from build123d import *

# Parameters (mm, degrees)
SKETCH_2_R                       = 28.3
EXTRUDE_1_DEPTH                  = 1.2
CUT_EXTRUDE_1_DEPTH              = 41.04022977
FILLET_1_R                       = 2
FILLET_2_R                       = 0.2
PATTERN_CIRCULAR_2_COUNT         = 6
FILLET_1_OF_PATTERN_CIRCULAR_2_R = 2
FILLET_2_OF_PATTERN_CIRCULAR_2_R = 0.2
SKETCH_4_R                       = 1.25
SKETCH_4_R_2                     = 1.5
CUT_EXTRUDE_2_DEPTH              = 40.283043416
CUT_EXTRUDE_START                = -1.2
CUT_EXTRUDE_4_DEPTH              = 1.2
SKETCH_7_W                       = 2.25
SKETCH_7_H                       = 2.05
EXTRUDE_2_DEPTH                  = 1.2
SKETCH_8_R                       = 1.3
CUT_EXTRUDE_6_DEPTH              = 1.2
CUT_EXTRUDE_7_DEPTH              = 1.2
FILLET_4_R                       = 1


with BuildPart() as part:
    # ｽｹｯﾁ2 → ﾎﾞｽ - 押し出し1 (new body)
    with BuildSketch(Plane.XY):
        Circle(SKETCH_2_R)
    extrude(amount=EXTRUDE_1_DEPTH)

    # ｽｹｯﾁ3 → ｶｯﾄ - 押し出し1 (cut, through all)
    with BuildSketch(Plane.XY.offset(1.2)):
        Polygon((-7.75, 30.775), (7.75, 30.775), (7.75, 24.3), (10, 24.3), (10, 22.25), (7.75, 22.25), (7.75, 15.775), (-7.75, 15.775), (-7.75, 22.25), (-10, 22.25), (-10, 24.3), (-7.75, 24.3), align=None)
    cut_extrude_1 = extrude(amount=-CUT_EXTRUDE_1_DEPTH, mode=Mode.SUBTRACT)

    # ﾌｨﾚｯﾄ1
    fillet_1_edges = [part.edges().sort_by_distance(p)[0] for p in [
        (7.75, 15.775, 0.6),
        (-7.75, 15.775, 0.6),
    ]]
    fillet(fillet_1_edges, radius=FILLET_1_R)

    # ﾌｨﾚｯﾄ2
    fillet_2_edges = [part.edges().sort_by_distance(p)[0] for p in [
        (-10, 22.25, 0.6),
        (-10, 24.3, 0.6),
        (10, 24.3, 0.6),
        (10, 22.25, 0.6),
    ]]
    fillet(fillet_2_edges, radius=FILLET_2_R)

    # 円形ﾊﾟﾀｰﾝ2: ｶｯﾄ - 押し出し1 ×6 about axis
    pattern_circular_2_axis = Axis((0, 0, 0), (0, 0, 1))
    for i in range(1, PATTERN_CIRCULAR_2_COUNT):
        add(cut_extrude_1.rotate(pattern_circular_2_axis, i * 360 / PATTERN_CIRCULAR_2_COUNT), mode=Mode.SUBTRACT)

    # ﾌｨﾚｯﾄ1 of 円形ﾊﾟﾀｰﾝ2
    fillet_1_of_pattern_circular_2_edges = [part.edges().sort_by_distance(p)[0] for p in [
        (-9.786550745, 14.599196879, 0.6),
        (-17.536550745, 1.175803121, 0.6),
        (-17.536550745, -1.175803121, 0.6),
        (-9.786550745, -14.599196879, 0.6),
        (-7.75, -15.775, 0.6),
        (7.75, -15.775, 0.6),
        (9.786550745, -14.599196879, 0.6),
        (17.536550745, -1.175803121, 0.6),
        (17.536550745, 1.175803121, 0.6),
        (9.786550745, 14.599196879, 0.6),
    ]]
    fillet(fillet_1_of_pattern_circular_2_edges, radius=FILLET_1_OF_PATTERN_CIRCULAR_2_R)

    # ﾌｨﾚｯﾄ2 of 円形ﾊﾟﾀｰﾝ2
    fillet_2_of_pattern_circular_2_edges = [part.edges().sort_by_distance(p)[0] for p in [
        (-24.269065234, 2.464745962, 0.6),
        (-26.044417312, 3.489745962, 0.6),
        (-16.044417312, 20.810254038, 0.6),
        (-14.269065234, 19.785254038, 0.6),
        (-14.269065234, -19.785254038, 0.6),
        (-16.044417312, -20.810254038, 0.6),
        (-26.044417312, -3.489745962, 0.6),
        (-24.269065234, -2.464745962, 0.6),
        (10, -22.25, 0.6),
        (10, -24.3, 0.6),
        (-10, -24.3, 0.6),
        (-10, -22.25, 0.6),
        (24.269065234, -2.464745962, 0.6),
        (26.044417312, -3.489745962, 0.6),
        (16.044417312, -20.810254038, 0.6),
        (14.269065234, -19.785254038, 0.6),
        (14.269065234, 19.785254038, 0.6),
        (16.044417312, 20.810254038, 0.6),
        (26.044417312, 3.489745962, 0.6),
        (24.269065234, 2.464745962, 0.6),
    ]]
    fillet(fillet_2_of_pattern_circular_2_edges, radius=FILLET_2_OF_PATTERN_CIRCULAR_2_R)

    # ｽｹｯﾁ4 → ｶｯﾄ - 押し出し2 (cut, through all)
    with BuildSketch(Plane.XY.offset(1.2)):
        with Locations((11.25, -19.485571585)):
            Circle(SKETCH_4_R)
        with Locations((11.25, -58.456714755)):
            Circle(SKETCH_4_R)
        with Locations((-22.5, -77.942286341)):
            Circle(SKETCH_4_R)
        with Locations((-56.25, -58.456714755)):
            Circle(SKETCH_4_R)
        with Locations((-56.25, -19.485571585)):
            Circle(SKETCH_4_R)
        with Locations((-22.5, 0)):
            Circle(SKETCH_4_R)
        with Locations((5.5, -9.526279442)):
            Circle(SKETCH_4_R_2)
        with Locations((-11, 0)):
            Circle(SKETCH_4_R_2)
        with Locations((5.5, 9.526279442)):
            Circle(SKETCH_4_R_2)
    extrude(amount=-CUT_EXTRUDE_2_DEPTH, mode=Mode.SUBTRACT)

    # ｽｹｯﾁ5 → ｶｯﾄ - 押し出し4 (cut)
    with BuildSketch(Plane.XY.offset(1.2).offset(CUT_EXTRUDE_START)):
        with BuildLine():
            Line((-19.69660633, 20.320770139), (-8.358999874, 13.775))
            Line((-8.358999874, 13.775), (8.358999874, 13.775))
            Line((8.358999874, 13.775), (19.69660633, 20.320770139))
            ThreePointArc((19.69660633, 20.320770139), (0, -28.3), (-19.69660633, 20.320770139))
        make_face()
    extrude(amount=CUT_EXTRUDE_4_DEPTH, mode=Mode.SUBTRACT)

    # ｽｹｯﾁ7 → ﾎﾞｽ - 押し出し2 (add)
    with BuildSketch(Plane.XY.offset(1.2)):
        Polygon((-17.169417312, 18.861696879), (-16.044417312, 20.810254038), (-14.269065234, 19.785254038), (-15.394065234, 17.836696879), align=None)
        Polygon((17.169417312, 18.861696879), (15.394065234, 17.836696879), (14.269065234, 19.785254038), (16.044417312, 20.810254038), align=None)
        with Locations((-8.875, 23.275)):
            Rectangle(SKETCH_7_W, SKETCH_7_H)
        with Locations((8.875, 23.275)):
            Rectangle(SKETCH_7_W, SKETCH_7_H)
    extrude(amount=-EXTRUDE_2_DEPTH)

    # ｽｹｯﾁ8 → ｶｯﾄ - 押し出し6 (cut)
    with BuildSketch(Plane.XY.offset(1.2)):
        with Locations((11.25, 19.485571585)):
            Circle(SKETCH_8_R)
        with Locations((-11.25, 19.485571585)):
            Circle(SKETCH_8_R)
    extrude(amount=-CUT_EXTRUDE_6_DEPTH, mode=Mode.SUBTRACT)

    # ｽｹｯﾁ9 → ｶｯﾄ - 押し出し7 (cut)
    with BuildSketch(Plane.XY.offset(1.2)):
        with BuildLine():
            ThreePointArc((0, 73.021527127), (68.160815364, 54.81940806), (0, 36.617288992))
            ThreePointArc((0, 36.617288992), (-68.160815364, 54.81940806), (0, 73.021527127))
        make_face()
    extrude(amount=-CUT_EXTRUDE_7_DEPTH, mode=Mode.SUBTRACT)

    # ﾌｨﾚｯﾄ4
    fillet_4_edges = [part.edges().sort_by_distance(p)[0] for p in [
        (19.69660633, 20.320770139, 0.6),
        (-19.69660633, 20.320770139, 0.6),
        (-7.75, 27.21814652, 0.6),
        (7.75, 27.21814652, 0.6),
    ]]
    fillet(fillet_4_edges, radius=FILLET_4_R)


solid = part.part
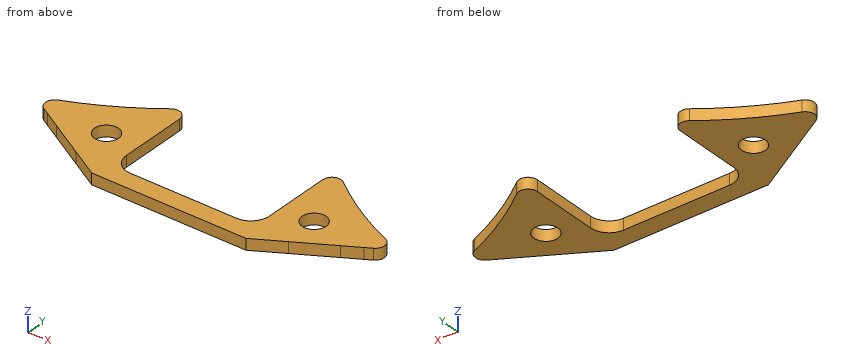
Model file for the job. Use its own axes, mm. Give positions to 0.01 mm unless a question says otherwise; leave off trailing zeros. Loops run counter-clockwise (first coordinate to the right, second up) from the corner with the lowest first, then second, coordinate; pieces in that order, holes last.
1) Wall check: line 1 (X direction, y = 24, z = 0.8); line 2 (X direction, y = 17.5, z = 0.95); line 3 (Y direction, x = 11.25, z = 0.95). Give the ranges that are in metal, low to high.
2) Saw through at A-A (y = 24.25). Write the cut outline in (x, z), plus the area to 3 significant figures.
3) Saw through at B-B (z = 1). Count the separate pieces of the cut face and the enclosed holes in it, plus the area to 3 significant figures.
4) Saw through at C-C (y = 16.75). Write the cut outline in (x, z), plus the area to 3 significant figures.
5) Saw through at D-D (x = -1.5). Write the cut outline in (y, z) (3 decimals), plus the area to 3 significant figures.
6) Flat gauge pins, fed straight in: pin 1 Ø3.5 at (x, y) = (-11.25, 19.49) entering from -Z; pin 2 Ø0.6 at (y, z) = (21.5, 0.5) entering from +X. Where does each tip first touch, or does it go through?
Answer block:
1. line 1: x = -12.07 to -7.75, 7.75 to 12.07
1. line 2: x = -14.81 to -7.73, 7.73 to 14.81
1. line 3: y = 15.44 to 18.19, 20.79 to 24.54
2. outline: (-11.69, 0) - (-7.75, 0) - (-7.75, 1.2) - (-11.69, 1.2) - close; (7.75, 0) - (11.69, 0) - (11.69, 1.2) - (7.75, 1.2) - close
2. area: 9.45 mm2
3. separate pieces: 1
3. enclosed holes: 2
3. area: 171 mm2
4. outline: (-13.51, 0) - (-7.47, 0) - (-7.47, 1.2) - (-13.51, 1.2) - close; (7.47, 0) - (13.51, 0) - (13.51, 1.2) - (7.47, 1.2) - close
4. area: 14.5 mm2
5. outline: (13.775, 0) - (15.775, 0) - (15.775, 1.2) - (13.775, 1.2) - close
5. area: 2.40 mm2
6. pin 1: stops at z = 0
6. pin 2: stops at x = 17.41
